Check sheet for the modelled part. Datum: model origin and axes. Units: mm. Round coordinates to 2 decimals unless told otherwise and drop trailing zeros. Write each loop counter-clockwise with the first axis right and the second up, starting at its lowest first coordinate (ties: lowest second). Pieces come first, ordered by that corner, then holes.
Item 1: Material ranges on line 1 along Z through (x, y) = (99, 0.6); line 2 along Z through (x, y) = (354, 0.9); line 3 along X through (y, z) = (1.5, -37), recorded low to high.
Item 2: Section check A-A, the plane y = 2.45. Record the cut outline in (x, z).
Item 3: Depth check by flat-ended pin: pin 1 (1 mm diameter, centred on x = 369, y = 0.5, fed in from -Z); pin 2 (1.5 mm diameter, centred on x = 87.5, y = 2.5, fed in from -Z). Enter the tip coordinate at first touch or a pass-through.
Item 4: Section check C-C, the plane z = -40.5. Record the cut outline in (x, y), plus the area to 3 significant figures.
Item 5: Section check B-B, the plane x = 436. Record the cut outline in (y, z).
from build123d import *

# Parameters (mm, degrees)
BOSS_EXTRU_1_DEPTH = 3


with BuildPart() as part:
    # Esquisse1 → Boss.-Extru.1 (new body)
    # profile 1 of 2: a face of its own
    with BuildSketch(Plane(origin=(0, 0, 0), x_dir=(1, 0, 0), z_dir=(0, 1, 0))):
        Polygon((103.757359313, 283), (165.248287591, 283), (468, 232.541381265), (468, 7), (113.757359313, 7), (32, 88.757359313), (32, 211.242640687), align=None)
        Polygon((105, 280), (165, 280), (465, 230), (465, 10), (115, 10), (35, 90), (35, 210), align=None, mode=Mode.SUBTRACT)
    # profile 2 of 2: a face of its own
    with BuildSketch(Plane(origin=(0, 0, 0), x_dir=(1, 0, 0), z_dir=(0, 1, 0))):
        Polygon((165, 280), (465, 230), (465, 10), (115, 10), (35, 90), (35, 210), (105, 280), align=None)
    extrude(amount=BOSS_EXTRU_1_DEPTH)


solid = part.part
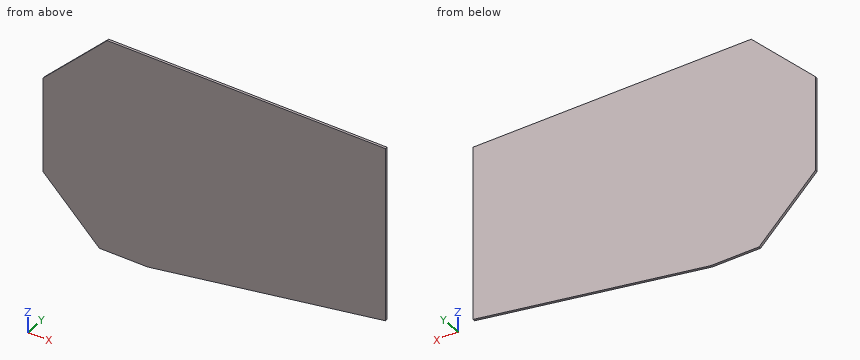
Values found:
1. line 1: z = -278.24 to -21.76
1. line 2: z = -251.54 to -7
1. line 3: x = 83.76 to 468
2. outline: (32, -211.24) - (103.76, -283) - (165.25, -283) - (468, -232.54) - (468, -7) - (113.76, -7) - (32, -88.76) - close
3. pin 1: stops at z = -249.12
3. pin 2: stops at z = -267.49
4. outline: (80.26, 0) - (468, 0) - (468, 3) - (80.26, 3) - close
4. area: 1,160 mm2
5. outline: (0, -237.87) - (3, -237.87) - (3, -7) - (0, -7) - close
